```python
from build123d import *

# Parameters (mm, degrees)
SKETCH1_R               = 1.75
SKETCH1_W               = 53
SKETCH1_H               = 30
BOSS_EXTRUDE1_DEPTH     = 2
BOSS_EXTRUDE2_OUTLINE_R = 1.75
BOSS_EXTRUDE2_DEPTH     = 11.5
SKETCH3_R               = 1.75
SKETCH3_W               = 53
SKETCH3_H               = 30
BOSS_EXTRUDE3_DEPTH     = 2
BOSS_EXTRUDE4_DEPTH     = 6
BOSS_EXTRUDE5_DEPTH     = 6
SKETCH7_W               = 3.3
SKETCH7_H               = 5
CUT_EXTRUDE3_DEPTH      = 2
SKETCH9_W               = 55
SKETCH9_H               = 5.5
CUT_EXTRUDE5_DEPTH      = 14
SKETCH10_W              = 5.5
SKETCH10_H              = 11.5
BOSS_EXTRUDE6_DEPTH     = 55
BOSS_EXTRUDE8_DEPTH     = 8.5
SKETCH14_R              = 1.25
CUT_EXTRUDE6_DEPTH      = 10


# Read off the part's stored shape, not the designer's step: Boss-Extrude2
with BuildPart() as part:
    # Sketch1 → Boss-Extrude1 (new body)
    with BuildSketch(Plane(origin=(0, 0, 0), x_dir=(1, 0, 0), z_dir=(0, 1, 0))):
        Polygon((0, 0), (23.2, 0), (23.2, -4.55), (20.8, -4.55), (20.8, -10), (28.65, -10), (28.65, -4.55), (71.7, -4.55), (71.7, 0), (83, 0), (83, -22.35), (83, -30.15), (83, -55), (72.2, -55), (72.2, -50.45), (33.2, -50.45), (33.2, -55), (0, -55), (0, -50.35), (19, -50.35), (19, -41.35), (0, -41.35), (0, -21.95), (17, -21.95), (17, -9.75), (0, -9.75), align=None)
        with Locations(Location((13.5, -4.85, 0), (0, 0, 270))):
            Circle(SKETCH1_R, mode=Mode.SUBTRACT)
        with Locations((47.3, -30.45)):
            Rectangle(SKETCH1_W, SKETCH1_H, mode=Mode.SUBTRACT)
    extrude(amount=BOSS_EXTRUDE1_DEPTH)

    # Boss-Extrude2 outline → Boss-Extrude2 (add)
    with BuildSketch(Plane.XZ):
        Polygon((0, 9.75), (0, 0), (20.8, 0), (20.8, 55), (0, 55), (0, 50.35), (19, 50.35), (19, 41.35), (0, 41.35), (0, 21.95), (17, 21.95), (17, 9.75), align=None)
        with Locations((13.5, 4.85)):
            Circle(BOSS_EXTRUDE2_OUTLINE_R, mode=Mode.SUBTRACT)
    extrude(amount=BOSS_EXTRUDE2_DEPTH)

    # Sketch3 → Boss-Extrude3 (add)
    with BuildSketch(Plane(origin=(0, 2, 0), x_dir=(1, 0, 0), z_dir=(0, 1, 0))):
        Polygon((23.2, 0), (0, 0), (0, -55), (33.2, -55), (33.2, -50.45), (72.2, -50.45), (72.2, -55), (83, -55), (83, 0), (71.7, 0), (71.7, -4.55), (28.65, -4.55), (28.65, -10), (20.8, -10), (20.8, -4.55), (23.2, -4.55), align=None)
        with Locations(Location((13.5, -4.85, 0), (0, 0, 90))):
            Circle(SKETCH3_R, mode=Mode.SUBTRACT)
        with Locations((47.3, -30.45)):
            Rectangle(SKETCH3_W, SKETCH3_H, mode=Mode.SUBTRACT)
    extrude(amount=BOSS_EXTRUDE3_DEPTH)

    # Sketch4 → Boss-Extrude4 (add)
    with BuildSketch(Plane.XY.offset(55)):
        Polygon((0, 4), (33.2, 4), (33.2, 0), (33.2, -1), (72.2, -1), (72.2, 0), (72.2, 4), (83, 4), (83, -11.5), (83, -16.5), (0, -16.5), (0, -11.5), align=None)
    extrude(amount=BOSS_EXTRUDE4_DEPTH)

    # Sketch5 → Boss-Extrude5 (add)
    with BuildSketch(Plane(origin=(0, 0, 0), x_dir=(-1, 0, 0), z_dir=(0, 0, -1))):
        Polygon((-23.2, 4), (-23.2, 0), (-23.2, -1), (-71.7, -1), (-71.7, 0), (-71.7, 4), (-83, 4), (-83, -11.5), (-83, -16.5), (0, -16.5), (0, -11.5), (0, 4), align=None)
    extrude(amount=BOSS_EXTRUDE5_DEPTH)

    # Sketch7 → Cut-Extrude3 (cut)
    with BuildSketch(Plane(origin=(0, 0, 55), x_dir=(-1, 0, 0), z_dir=(0, 0, -1))):
        with Locations((-14.15, -14)):
            Rectangle(SKETCH7_W, SKETCH7_H)
        with Locations((-68.85, -14)):
            Rectangle(SKETCH7_W, SKETCH7_H)
    extrude(amount=-CUT_EXTRUDE3_DEPTH, mode=Mode.SUBTRACT)

    # Sketch9 → Cut-Extrude5 (cut)
    with BuildSketch(Plane(origin=(20.8, 0, 0), x_dir=(0, 0, -1), z_dir=(1, 0, 0))):
        with Locations((-27.5, -8.75)):
            Rectangle(SKETCH9_W, SKETCH9_H)
    extrude(amount=-CUT_EXTRUDE5_DEPTH, mode=Mode.SUBTRACT)

    # Sketch10 → Boss-Extrude6 (add)
    with BuildSketch(Plane(origin=(0, 0, 55), x_dir=(-1, 0, 0), z_dir=(0, 0, -1))):
        with Locations((-80.25, -5.75)):
            Rectangle(SKETCH10_W, SKETCH10_H)
    extrude(amount=BOSS_EXTRUDE6_DEPTH)

    # Sketch12 → Boss-Extrude8 (add)
    with BuildSketch(Plane.XZ):
        Polygon((73.8, 45.45), (77.5, 45.45), (77.5, 50.45), (72.2, 50.45), (36.8, 50.45), (36.8, 45.45), align=None)
        Polygon((28.65, 10), (28.65, 4.55), (71.7, 4.55), (77.5, 4.55), (77.5, 15.45), (73.8, 15.45), (28.65, 15.45), align=None)
    extrude(amount=BOSS_EXTRUDE8_DEPTH)

    # Sketch14 → Cut-Extrude6 (cut)
    with BuildSketch(Plane.XZ.offset(16.5)):
        with Locations(Location((5, 58, 0), (0, 0, 270))):
            Circle(SKETCH14_R)
        with Locations(Location((78, 58, 0), (0, 0, 90))):
            Circle(SKETCH14_R)
        with Locations(Location((78, -3, 0), (0, 0, 270))):
            Circle(SKETCH14_R)
        with Locations(Location((5, -3, 0), (0, 0, 90))):
            Circle(SKETCH14_R)
    extrude(amount=-CUT_EXTRUDE6_DEPTH, mode=Mode.SUBTRACT)


solid = part.part
```
Check sheet for the modelled part. Datum: model origin and axes. Units: mm. A direction names the side the tool comes from. Round coordinates to 2 decimals unless told otherwise and drop trailing zeros. Loops run counter-clockwise (first coordinate to the right, second up) from the corner with the lowest first, then second, coordinate; pieces in that order, holes last. Notation, with made-up numbers: (73.25, 83) -> (123.25, 83) arc R29 ccw to (123.25, 120) -> close; hole circle Ø2 at (23.5, -33.75). An arc over 180 degrees is marked (long way). Write item = value, one per line. Start each with the question number.
1) Set-up check for faces 1 (the flat face through (42, -16.5, 58)), 2 (the flat face through (29, 0, 50)), 3 (the flat face through (80, -11.5, 28)), 4 (the flat face through (9, 2, 46)): record each of +Z, -Z, +X, -X, +Y, -Y from which the full face is reachable in a straight line by a thin tool's end or side.
2) Sectioned sample at C-C, the plane z = 37.5. Record the cut outline in (x, y), plus the area to 3 significant figures.
3) Release check for a two-part mould opening along Z. For faces 5 (the flat face through (83, -4, 28)), 6 (the flat face through (42, -8, -6)), 7 (the flat face through (7, -3, 9.75)) record: released by +Z, released by -Z, zero draft, split by the parting line, or undercut.
4) Sectioned sample at B-B, the plane x = 13.5. Record the cut outline in (y, z), plus the area to 3 significant figures.
5) Thickness scan on probe 1 along X at (y, z) = (2.5, 4.85); probe 2 along Z at (x, y) = (78, -12); probe 3 along Z at (x, y) = (55.5, -2.5). Record the ranges inside material, lowest first.
6) Sectioned sample at D-D, the plane y = -2.75. Record the cut outline in (x, z).
7) Sectioned sample at A-A, the plane y = -14.25. Record the cut outline in (x, z).
8) Gauge pin test, flat ends, axial feed: pin 1 Ø7 at (x, z) = (11, 44) entering from -Y; pin 2 Ø3 at (y, z) = (-14, 8) entering from +X; pin 3 Ø2 at (x, z) = (3, 27) entering from -Y; pin 4 Ø2.5 at (x, z) = (26, 13.5) entering from -Y. Record the tip position at first contact, or that the pin passes through.
Results are:
q1.face_1 = +Z, -Z, +X, -X, -Y
q1.face_2 = -Y
q1.face_3 = +X, -X, -Y
q1.face_4 = -X, -Y
q2.outline = (0, -11.5) -> (6.8, -11.5) -> (6.8, -6) -> (20.8, -6) -> (20.8, 4) -> (0, 4) -> close; (73.8, 0) -> (77.5, 0) -> (77.5, -11.5) -> (83, -11.5) -> (83, 4) -> (73.8, 4) -> close
q2.area = 345 mm^2
q3.face_5 = zero draft
q3.face_6 = released by -Z
q3.face_7 = undercut
q4.outline = (-16.5, -6) -> (4, -6) -> (4, 3.1) -> (-6, 3.1) -> (-6, 0) -> (-16.5, 0) -> close; (-16.5, 57) -> (-11.5, 57) -> (-11.5, 55) -> (-6, 55) -> (-6, 50.35) -> (2, 50.35) -> (2, 41.35) -> (-6, 41.35) -> (-6, 21.95) -> (2, 21.95) -> (2, 9.75) -> (-6, 9.75) -> (-6, 6.6) -> (4, 6.6) -> (4, 61) -> (-16.5, 61) -> close
q4.area = 581 mm^2
q5.probe_1 = 0 to 11.75, 15.25 to 20.8, 28.65 to 83
q5.probe_2 = -6 to -4.25, -1.75 to 0, 55 to 56.75, 59.25 to 61
q5.probe_3 = -6 to 0, 4.55 to 15.45, 45.45 to 50.45, 55 to 61
q6.outline = (0, -6) -> (83, -6) -> (83, 61) -> (0, 61) -> (0, 50.35) -> (19, 50.35) -> (19, 41.35) -> (0, 41.35) -> (0, 21.95) -> (17, 21.95) -> (17, 9.75) -> (0, 9.75) -> close; hole circle Ø3.5 at (13.5, 4.85); hole (20.8, 0) -> (77.5, 0) -> (77.5, 4.55) -> (28.65, 4.55) -> (28.65, 15.45) -> (77.5, 15.45) -> (77.5, 45.45) -> (36.8, 45.45) -> (36.8, 50.45) -> (77.5, 50.45) -> (77.5, 55) -> (20.8, 55) -> close
q7.outline = (0, -6) -> (83, -6) -> (83, 0) -> (0, 0) -> close; (0, 55) -> (12.5, 55) -> (12.5, 57) -> (15.8, 57) -> (15.8, 55) -> (67.2, 55) -> (67.2, 57) -> (70.5, 57) -> (70.5, 55) -> (83, 55) -> (83, 61) -> (0, 61) -> close; hole circle Ø2.5 at (5, -3); hole circle Ø2.5 at (5, 58); hole circle Ø2.5 at (78, -3); hole circle Ø2.5 at (78, 58)
q8.pin_1 = -6
q8.pin_2 = through
q8.pin_3 = -11.5
q8.pin_4 = 0
